```python
from build123d import *

# Parameters (mm, degrees)
SKETCH_1_W          = 14.1
SKETCH_1_H          = 12
EXTRUDE_1_DEPTH     = 11
SKETCH_2_W          = 1.5
SKETCH_2_H          = 12
CUT_EXTRUDE_1_DEPTH = 1.8
SKETCH_3_W          = 9
SKETCH_3_H          = 12
CUT_EXTRUDE_2_DEPTH = 1.8
EXTRUDE_2_DEPTH     = 9
SKETCH_5_W          = 1
SKETCH_5_H          = 2
CUT_EXTRUDE_3_DEPTH = 12


with BuildPart() as part:
    # Эскиз1 → Бобышка-Вытянуть1 (new body)
    with BuildSketch(Plane.XY):
        with Locations((4.962698413, 0.73968254)):
            Rectangle(SKETCH_1_W, SKETCH_1_H)
    extrude_1 = extrude(amount=EXTRUDE_1_DEPTH)

    # Эскиз2 → Вырез-Вытянуть1 (cut)
    with BuildSketch(Plane(origin=(0, 0, 0), x_dir=(-1, 0, 0), z_dir=(0, 0, -1))):
        with Locations((-0.662698413, 0.73968254)):
            Rectangle(SKETCH_2_W, SKETCH_2_H)
    cut_extrude_1 = extrude(amount=-CUT_EXTRUDE_1_DEPTH, mode=Mode.SUBTRACT)

    # Эскиз3 → Вырез-Вытянуть2 (cut)
    with BuildSketch(Plane(origin=(0, 0, 0), x_dir=(-1, 0, 0), z_dir=(0, 0, -1))):
        with Locations((-7.512698413, 0.73968254)):
            Rectangle(SKETCH_3_W, SKETCH_3_H)
    cut_extrude_2 = extrude(amount=-CUT_EXTRUDE_2_DEPTH, mode=Mode.SUBTRACT)

    # Эскиз4 → Бобышка-Вытянуть2 (add)
    with BuildSketch(Plane(origin=(12.012698413, 0, 0), x_dir=(0, 0, -1), z_dir=(1, 0, 0))):
        Polygon((-1.8, -5.26031746), (-0.4, -5.26031746), (-1.8, -3.86031746), align=None)
    extrude_2 = extrude(amount=-EXTRUDE_2_DEPTH)

    # Эскиз5 → Вырез-Вытянуть3 (cut)
    with BuildSketch(Plane(origin=(12.012698413, 0, 0), x_dir=(0, 0, -1), z_dir=(1, 0, 0))):
        with Locations((-10.5, -4.26031746)):
            Rectangle(SKETCH_5_W, SKETCH_5_H)
    cut_extrude_3 = extrude(amount=-CUT_EXTRUDE_3_DEPTH, mode=Mode.SUBTRACT)

    # Зеркальное отражение1: Бобышка-Вытянуть1, Вырез-Вытянуть1, Вырез-Вытянуть2, Бобышка-Вытянуть2, Вырез-Вытянуть3 across plane
    add(extrude_1.mirror(Plane.XY.offset(11)))
    add(cut_extrude_1.mirror(Plane.XY.offset(11)), mode=Mode.SUBTRACT)
    add(cut_extrude_2.mirror(Plane.XY.offset(11)), mode=Mode.SUBTRACT)
    add(extrude_2.mirror(Plane.XY.offset(11)))
    add(cut_extrude_3.mirror(Plane.XY.offset(11)), mode=Mode.SUBTRACT)


solid = part.part
```
Part model, mm, in its own coordinate system. A direction names the side the tool comes from. Coordinates: 2 decimals unless noted, no trailing zeros. Loops run counter-clockwise (first coordinate to the right, second up) from the corner with the lowest first, then second, coordinate; pieces in that order, holes last. Notation, with made-up numbers: (7, -36.5) - (28, -36.5) arc R25 ccw to (28, -10.5) - close; hole circle Ø9 at (12, 76). An arc over 180 degrees is marked (long way). Write item = value, one per line. Start each with the question number.
Item 1: 3-axis set-ups, long thin cutter, end or side, ignore diameter. For faces 1 (the flat face through (1.413, 1, 1)), 2 (the flat face through (3.013, 1, 1)), 3 (the flat face through (3.013, 1, 21)), 4 (the flat face through (0.013, -4, 11)): which of +Z, -Z, +X, -X, +Y, -Y reach the whole face in a straight line?
Item 2: Cut at C-C, the plane z = 10.25. Give the cut face in (x, y), and give its area (3 significant figures).
Item 3: Flat gauge pins, fed straight in: pin 1 Ø5 at (x, y) = (10.5, 3) entering from +Z; pin 2 Ø0.9 at (y, z) = (0.5, 0.5) entering from +X; pin 3 Ø2 at (y, z) = (-4.5, 10.5) entering from +X; pin 4 Ø1.6 at (x, y) = (6, -4) entering from -Z. Where does each tip first touch, or does it go through?
Item 4: Mould opens along Z. For faces 5 (the flat face through (-2.087, 1, 11)), 6 (the flat face through (6, -3.26, 11)), 7 (the flat face through (8, 2, 1.8)), 8 (the flat face through (7.58, -4.57, 20.91)) say: released by +Z, released by -Z, zero draft, split by the parting line, or undercut.
Item 5: Cut at D-D, the plane y = -3.5. Give the cut face in (x, z), and give its area (3 significant figures).
Item 6: Cut at A-A, the plane y = -0.5. Give the cut face in (x, z).
Item 7: Cut at B-B, the plane x = 9.25. Give the cut face in (y, z), and give its area (3 significant figures).
Item 8: Wall check: L1, parallel to X at y = -2, z = 20.25; L2, parallel to Z at x = 7.5, y = -1; L3, parallel to Y at x = 6.75, z = 10.75. Give the ranges that are in metal, low to high. Write a range as from..to.
The answers:
q1.face_1 = -Z, +Y, -Y
q1.face_2 = -Z, +X, +Y
q1.face_3 = +Z, +X, +Y
q1.face_4 = +X, -Y
q2.outline = (-2.09, -5.26) - (0.01, -5.26) - (0.01, -3.26) - (12.01, -3.26) - (12.01, 6.74) - (-2.09, 6.74) - close
q2.area = 145 mm2
q3.pin_1 = 20.2
q3.pin_2 = 3.01
q3.pin_3 = 12.01
q3.pin_4 = 0.86
q4.face_5 = zero draft
q4.face_6 = undercut
q4.face_7 = released by -Z
q4.face_8 = released by +Z
q5.outline = (-2.09, 0) - (-0.09, 0) - (-0.09, 1.8) - (1.41, 1.8) - (1.41, 0) - (3.01, 0) - (3.01, 1.8) - (12.01, 1.8) - (12.01, 10) - (0.01, 10) - (0.01, 12) - (12.01, 12) - (12.01, 20.2) - (3.01, 20.2) - (3.01, 22) - (1.41, 22) - (1.41, 20.2) - (-0.09, 20.2) - (-0.09, 22) - (-2.09, 22) - close
q5.area = 248 mm2
q6.outline = (-2.09, 0) - (-0.09, 0) - (-0.09, 1.8) - (1.41, 1.8) - (1.41, 0) - (3.01, 0) - (3.01, 1.8) - (12.01, 1.8) - (12.01, 20.2) - (3.01, 20.2) - (3.01, 22) - (1.41, 22) - (1.41, 20.2) - (-0.09, 20.2) - (-0.09, 22) - (-2.09, 22) - close
q7.outline = (-5.26, 0.4) - (-3.86, 1.8) - (6.74, 1.8) - (6.74, 20.2) - (-3.86, 20.2) - (-5.26, 21.6) - (-5.26, 12) - (-3.26, 12) - (-3.26, 10) - (-5.26, 10) - close
q7.area = 219 mm2
q8.L1 = -2.09..-0.09, 1.41..3.01
q8.L2 = 1.8..20.2
q8.L3 = -3.26..6.74
